from build123d import *

# Parameters (mm, degrees)
SKETCH1_R             = 25.4
SKETCH1_R_2           = 8.763
BOSS_EXTRUDE1_DEPTH   = 3.175
F_8_CLEARANCE_HOLE1_D = 4.4958


with BuildPart() as part:
    # Sketch1 → Boss-Extrude1 (new body)
    with BuildSketch(Plane(origin=(0, 0, 0), x_dir=(1, 0, 0), z_dir=(0, 1, 0))):
        Circle(SKETCH1_R)
        Circle(SKETCH1_R_2, mode=Mode.SUBTRACT)
    extrude(amount=BOSS_EXTRUDE1_DEPTH)

    # #8 Clearance Hole1 (through all)
    with Locations(Plane(origin=(0, 3.175, 0), x_dir=(1, 0, 0), z_dir=(0, 1, 0))):
        with Locations((13.97, 0), (0, 13.97), (-13.97, 0), (0, -13.97)):
            Hole(F_8_CLEARANCE_HOLE1_D / 2)


solid = part.part
CAD build for the part. Positions are in the model's coordinates, mm. Coordinates: 2 decimals unless noted, no trailing zeros. Loops run counter-clockwise (first coordinate to the right, second up) from the corner with the lowest first, then second, coordinate; pieces in that order, holes last. Notation, with made-up numbers: (-29.5, 9.5) - (4.5, 9.5) arc R29 cw to (4.5, 45.5) - close; hole circle Ø6 at (-25, 24.25). An arc over 180 degrees is marked (long way). Write item = value, one per line. Start each with the question number.
Q1. Cut at B-B, the plane x = 0. List the corners of the cut face in (y, z) (3 decimals), then the cut area to 3 significant figures.
Q2. Cut at C-C, the plane y = 2.65. List the corners of the cut face in (x, z), then the cut area to 3 significant figures.
Q3. Drill centre lines: L1, parallel to Z at x = 0, y = 0.7; L2, parallel to Z at x = -0.5, y = 2.55; L3, parallel to Z at x = -4, y = 0.8. Where is each one in solid material? Low to high.
Q4. Cut at D-D, the plane z = 8. List the corners of the cut face in (x, y) (3 decimals).
Q5. Pull direction X, two halves, no side cores. Call faces 1 (the flat face through (11, 3.175, 0)), 2 (the cylindrical face through (11.826, 1.565, -0.675)), 3 (the cylindrical face through (-5.506, 1.565, 24.796)): pulls with the +X half, pulls with the -X half, needs draft (parallel to the pull), parting line crosses it, or undercut.
Q6. Cut at A-A, the plane z = 0. List the corners of the cut face in (x, y) (3 decimals).
Computed:
q1.outline = (0, -25.4) - (3.175, -25.4) - (3.175, -16.218) - (0, -16.218) - close; (0, -11.722) - (3.175, -11.722) - (3.175, -8.763) - (0, -8.763) - close; (0, 8.763) - (3.175, 8.763) - (3.175, 11.722) - (0, 11.722) - close; (0, 16.218) - (3.175, 16.218) - (3.175, 25.4) - (0, 25.4) - close
q1.area = 77.1 mm²
q2.outline = circle Ø50.8 at (0, 0); hole circle Ø4.5 at (-13.97, 0); hole circle Ø17.53 at (0, 0); hole circle Ø4.5 at (0, -13.97); hole circle Ø4.5 at (0, 13.97); hole circle Ø4.5 at (13.97, 0)
q2.area = 1,720 mm²
q3.L1 = -25.4 to -16.22, -11.72 to -8.76, 8.76 to 11.72, 16.22 to 25.4
q3.L2 = -25.4 to -16.16, -11.78 to -8.75, 8.75 to 11.78, 16.16 to 25.4
q3.L3 = -25.08 to -7.8, 7.8 to 25.08
q4.outline = (-24.107, 0) - (-3.576, 0) - (-3.576, 3.175) - (-24.107, 3.175) - close; (3.576, 0) - (24.107, 0) - (24.107, 3.175) - (3.576, 3.175) - close
q5.face_1 = needs draft
q5.face_2 = undercut
q5.face_3 = parting line crosses it
q6.outline = (-25.4, 0) - (-16.218, 0) - (-16.218, 3.175) - (-25.4, 3.175) - close; (-11.722, 0) - (-8.763, 0) - (-8.763, 3.175) - (-11.722, 3.175) - close; (8.763, 0) - (11.722, 0) - (11.722, 3.175) - (8.763, 3.175) - close; (16.218, 0) - (25.4, 0) - (25.4, 3.175) - (16.218, 3.175) - close
